```python
from build123d import *

# Parameters (mm, degrees)
SKETCH1_R           = 4.4
SKETCH1_R_2         = 3.1
BOSS_EXTRUDE1_DEPTH = 6
BOSS_EXTRUDE2_DEPTH = 3
FILLET1_R           = 1


with BuildPart() as part:
    # Sketch1 → Boss-Extrude1 (new body)
    with BuildSketch(Plane.XY):
        with Locations((0, -3.7)):
            Circle(SKETCH1_R)
        with Locations((0, -3.7)):
            Circle(SKETCH1_R_2, mode=Mode.SUBTRACT)
    extrude(amount=-BOSS_EXTRUDE1_DEPTH)

    # Sketch2 → Boss-Extrude2 (add)
    with BuildSketch(Plane.XY):
        Polygon((9.815203288, -8.1), (9.815203288, 0.7), (-9.815203288, 0.7), (-9.815203288, 3.629197365), (-17.779678307, -3.7), (-9.815203288, -12.354817051), (-9.815203288, -8.1), align=None)
    extrude(amount=BOSS_EXTRUDE2_DEPTH)

    # Fillet1
    fillet1_edges = [part.edges().sort_by_distance(p)[0] for p in [
        (-13.797440798, -8.027408526, 0),
        (-17.779678307, -3.7, 1.5),
        (9.815203288, -8.1, 1.5),
        (9.815203288, 0.7, 1.5),
        (-13.797440798, -0.035401317, 0),
        (-13.797440798, -8.027408526, 3),
        (0, -8.1, 3),
        (9.815203288, -3.7, 3),
        (0, 0.7, 3),
        (-13.797440798, -0.035401317, 3),
    ]]
    fillet(fillet1_edges, radius=FILLET1_R)


solid = part.part
```
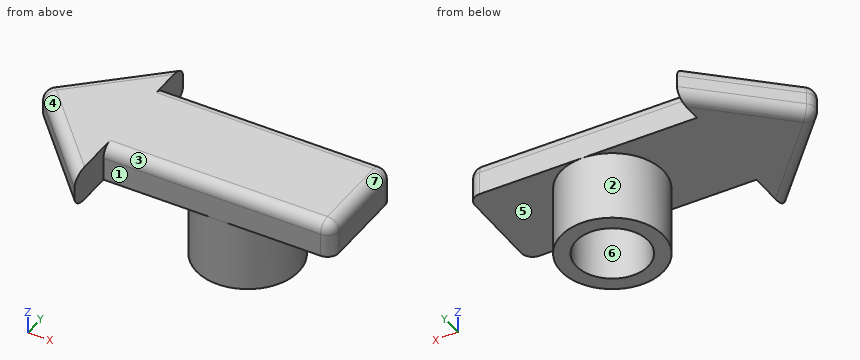
Here's how the part is built. I have some questions about the finished solid (model axes, mm). Face numbers are marked on the shaded views. A direction names the side the tool comes from. Give positions to 0.01 mm unless a question says otherwise; leave off trailing zeros. Write each loop counter-clockwise with the first axis right and the second up, starting at its lowest first coordinate (ties: lowest second). Pieces come first, ordered by that corner, then holes.
(1) Imagine slicing it at B-B, the plane z = -2. Write out the boundary of the cut face in (x, y).
Output values:
outline: circle Ø8.8 at (0, -3.7); hole circle Ø6.2 at (0, -3.7)
(2) Thinking about a two-plate mould opening in X: for the marked faces 4, 5, 6 and 7, which applies, pulls with the +X half, pulls with the -X half, needs draft (parallel to the pull), parting line crosses it, or undercut?
Output values:
face 4: pulls with the -X half
face 5: needs draft
face 6: undercut
face 7: pulls with the +X half
(3) Will these pins go through, and if not, where does the flat tip stop? pin 1 (2 mm diameter, centred on x = 2.5, z = -4.5, fed in from +Y); pin 2 (4 mm diameter, centred on x = -6.5, y = -1.5, fed in from -Z); pin 3 (3 mm diameter, centred on x = 1, z = -0.5, fed in from -Y).
Output values:
pin 1: stops at y = 0.44
pin 2: stops at z = 0
pin 3: stops at y = -8.1
(4) If I drill on L1, parallel to Y at x = 0, z = -4.35; L2, parallel to Z at x = 2.25, y = -4.75; L3, parallel to Y at x = -1.25, z = -4.5, over which ranges is the centre line in solid material (lowest first)?
Output values:
L1: y = -8.1 to -6.8, -0.6 to 0.7
L2: z = 0 to 3
L3: y = -7.92 to -6.54, -0.86 to 0.52
(5) Imagine slicing it at D-D, the plane x = 1.25. Write out the boundary of the cut face in (y, z), and give its area (3 significant figures).
Output values:
outline: (-8.1, 0) - (-7.92, 0) - (-7.92, -6) - (-6.54, -6) - (-6.54, 0) - (-0.86, 0) - (-0.86, -6) - (0.52, -6) - (0.52, 0) - (0.7, 0) - (0.7, 2) arc R1 ccw to (-0.3, 3) - (-7.1, 3) arc R1 ccw to (-8.1, 2) - close
area: 42.6 mm2
(6) On a 3-axis mill with a long thin cutter (end or side, diameter ignored), from which of +Z, -Z, +X, -X, +Y, -Y can I reach the whole of each face in a straight line? I mean the marked faces 1, 2 and 3. Say none if no direction works.
Output values:
face 1: +Z, -Z, +X, -Y
face 2: -Z
face 3: +Z, +X, -Y
(7) Imagine slicing it at A-A, the plane x = 8. Write out the boundary of the cut face in (y, z).
Output values:
outline: (-8.1, 0) - (0.7, 0) - (0.7, 2) arc R1 ccw to (-0.3, 3) - (-7.1, 3) arc R1 ccw to (-8.1, 2) - close
(8) Imagine slicing it at C-C, the plane x = -2.75. Write out the boundary of the cut face in (y, z), and give its area (3 significant figures).
Output values:
outline: (-8.1, 0) - (-7.13, 0) - (-7.13, -6) - (-5.13, -6) - (-5.13, 0) - (-2.27, 0) - (-2.27, -6) - (-0.27, -6) - (-0.27, 0) - (0.7, 0) - (0.7, 2) arc R1 ccw to (-0.3, 3) - (-7.1, 3) arc R1 ccw to (-8.1, 2) - close
area: 50.0 mm2
